Model file for the job. Use its own axes, mm. Round coordinates to 2 decimals unless told otherwise and drop trailing zeros. Order: outer loops, then holes, each group sorted by start corner. A loop starts at its lowest first (then second) coordinate and runs counter-clockwise, first axis right, second up. Notation, with made-up numbers: (-17.5, 15) -> (7.5, 15) arc R13 cw to (7.5, 25) -> close; hole circle Ø1 at (55.25, -5.75). An arc over 180 degrees is marked (long way). Put each result on its own line as item: value. Start each with the question number.
Q1. Cut at C-C, the plane z = 3. State how many separate pieces and enclosed holes the cut face has, and give its area (3 significant figures).
Q2. Flat gauge pin, fed straight in: P1, Ø2.5, axis at x = 102, y = 76.49, coming from the -Z side. Where does the tip first touch, or does it go through?
Q3. Probe L1, parallel to X at y = 64, z = 1.3; L2, parallel to Y at x = -2, z = 1.7; L3, parallel to X at y = 75, z = 0.3. List the from-to ranges inside material, lowest first.
Q4. Cut at A-A, the plane y = 51.5. List the corners of the cut face in (x, z), and give its area (3 significant figures).
Q5. Cut at B-B, the plane x = -23. List the corners of the cut face in (y, z).
from build123d import *

# Parameters (mm, degrees)
ESQUISSE1_W             = 145
ESQUISSE1_H             = 145
BOSS_EXTRU_1_DEPTH      = 5
ESQUISSE3_W             = 4
ESQUISSE3_H             = 20
ENL_V_MAT_EXTRU_1_DEPTH = 5
ESQUISSE2_R             = 2
ENL_V_MAT_EXTRU_2_DEPTH = 5


with BuildPart() as part:
    # Esquisse1 → Boss.-Extru.1 (new body)
    with BuildSketch(Plane.XY):
        with Locations((39.504598951, 13.991761527)):
            Rectangle(ESQUISSE1_W, ESQUISSE1_H)
    extrude(amount=BOSS_EXTRU_1_DEPTH)

    # Esquisse3 → Enlèv. mat.-Extru.1 (cut)
    with BuildSketch(Plane.XY.offset(5)):
        with Locations((79.604598951, 58.941761527)):
            Rectangle(ESQUISSE3_W, ESQUISSE3_H)
        with Locations((-0.595401049, 58.941761527)):
            Rectangle(ESQUISSE3_W, ESQUISSE3_H)
        with Locations((-0.595401049, -30.958238473)):
            Rectangle(ESQUISSE3_W, ESQUISSE3_H)
        with Locations((79.604598951, -30.958238473)):
            Rectangle(ESQUISSE3_W, ESQUISSE3_H)
    extrude(amount=-ENL_V_MAT_EXTRU_1_DEPTH, mode=Mode.SUBTRACT)

    # Esquisse2 → Enlèv. mat.-Extru.2 (cut)
    with BuildSketch(Plane.XY.offset(5)):
        with Locations((-22.995401049, 76.491761527)):
            Circle(ESQUISSE2_R)
        with Locations((102.004598951, 76.491761527)):
            Circle(ESQUISSE2_R)
        with Locations((102.004598951, -48.508238473)):
            Circle(ESQUISSE2_R)
        with Locations((-22.995401049, -48.508238473)):
            Circle(ESQUISSE2_R)
    extrude(amount=-ENL_V_MAT_EXTRU_2_DEPTH, mode=Mode.SUBTRACT)


solid = part.part
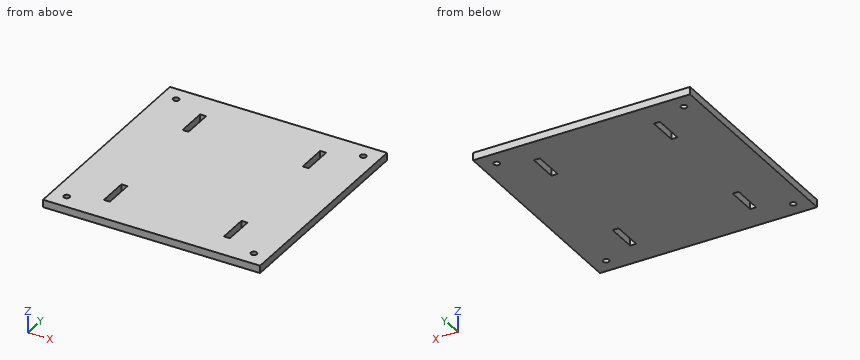
Ans:
1. separate pieces: 1
1. enclosed holes: 8
1. area: 20,700 mm^2
2. P1: passes through
3. L1: x = -33 to -2.6, 1.4 to 77.6, 81.6 to 112
3. L2: y = -58.51 to -40.96, -20.96 to 48.94, 68.94 to 86.49
3. L3: x = -33 to -24.33, -21.66 to 100.67, 103.34 to 112
4. outline: (-33, 0) -> (-2.6, 0) -> (-2.6, 5) -> (-33, 5) -> close; (1.4, 0) -> (77.6, 0) -> (77.6, 5) -> (1.4, 5) -> close; (81.6, 0) -> (112, 0) -> (112, 5) -> (81.6, 5) -> close
4. area: 685 mm^2
5. outline: (-58.51, 0) -> (-50.51, 0) -> (-50.51, 5) -> (-58.51, 5) -> close; (-46.51, 0) -> (74.49, 0) -> (74.49, 5) -> (-46.51, 5) -> close; (78.49, 0) -> (86.49, 0) -> (86.49, 5) -> (78.49, 5) -> close
